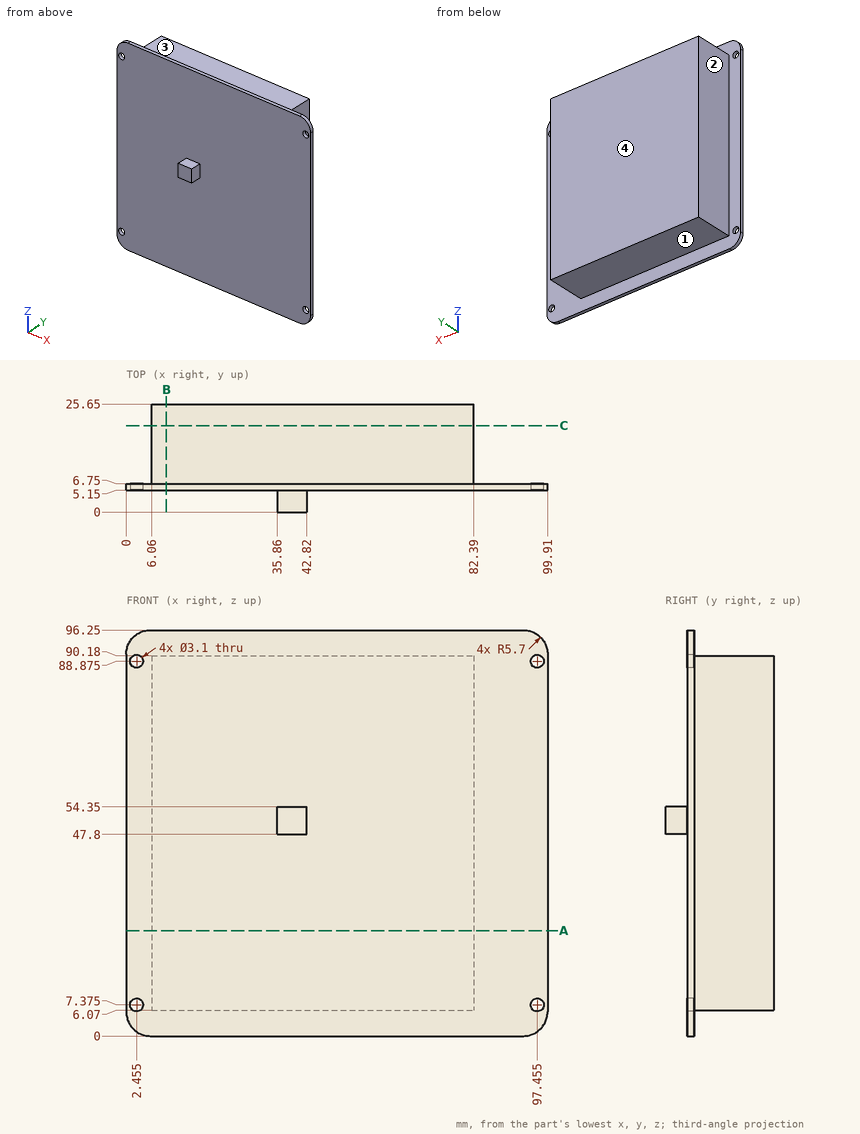
Answer from the drawing. Dimensions are ordinates in mm from the lowest x, y and z of the part. A direction names the side the tool comes from. Give positions to 0.01 mm unless a question says otherwise; leave off trailing zeros. Order: outer loops, then holes, each group sorted by start corner. A loop starts at its lowest first (then second) coordinate and runs counter-clockwise, first axis right, second up. Notation, with made-up numbers: (74, 10) -> (94, 10) arc R27 cw to (94, 29) -> close; hole circle Ø10 at (-15, -34). An arc over 180 degrees is marked (long way). One line per item, written item: value. Start each with the question number.
(1) Flat-ended cylindrical pins translate along their axes: P1, Ø5.5, axis at y = 15, z = 42.5, coming from the -X side; P2, Ø5.5, axis at x = 43.5, y = 14, coming from the -Z side; P3, Ø5.5, axis at x = 39.5, y = 1.5, coming from the -Z side. Find the tip coordinate at first contact, or state that the pin passes through.
(2) The part is cut by section C-C (y = 20.5). Determine the outline of the cut face in (x, z).
(3) Straight lines are drawn through the part: L1, parallel to X at y = 23.75, z = 7; L2, parallel to Y at x = 50, z = 12.5; L3, parallel to Z at x = 54, y = 16.5. For each, find the intervals that lie inside material, in ascending order.
(4) The part is cut by section A-A (z = 25). Determine the outline of the cut face in (x, y), and give its area (3 significant figures).
(5) The part is cut by section B-B (x = 9.5). Determine the outline of the cut face in (y, z).
(6) A tool of negligible diameter and unlimited length cuts with its end or side. For the marked faces 1, 2, 3 and 4, from which of +Z, -Z, +X, -X, +Y, -Y can it reach the whole face along a straight path? Write none if from no direction.
Taken from the geometry:
1. P1: x = 6.06
1. P2: z = 6.07
1. P3: z = 47.8
2. outline: (6.06, 6.07) -> (82.39, 6.07) -> (82.39, 90.18) -> (6.06, 90.18) -> close
3. L1: 6.06 to 82.39
3. L2: 5.15 to 25.65
3. L3: 6.07 to 90.18
4. outline: (0, 5.15) -> (99.91, 5.15) -> (99.91, 6.75) -> (82.39, 6.75) -> (82.39, 25.65) -> (6.06, 25.65) -> (6.06, 6.75) -> (0, 6.75) -> close
4. area: 1,600 mm^2
5. outline: (5.15, 0) -> (6.75, 0) -> (6.75, 6.07) -> (25.65, 6.07) -> (25.65, 90.18) -> (6.75, 90.18) -> (6.75, 96.25) -> (5.15, 96.25) -> close
6. face 1: -Z, +X, -X, +Y
6. face 2: +Z, -Z, -X, +Y
6. face 3: +Z, +X, -X, +Y
6. face 4: +Z, -Z, +X, -X, +Y
